Geometry: see drawing. Coordinates: mm, zero at the bounding-box minimum. Round coordinates to 2 decimals unless told otherwise and drop trailing zeros. Loops run counter-clockwise (first coordinate to the right, second up) from the corner with the lowest first, then second, coordinate; pieces in that order, holes last. Notation, with made-up numbers: (0.25, 74) -> (5.25, 74) arc R26 cw to (5.25, 100) -> close; hole circle Ø9 at (55, -37). An arc over 180 degrees is marked (long way). Answer in a Markdown table with one row per item.
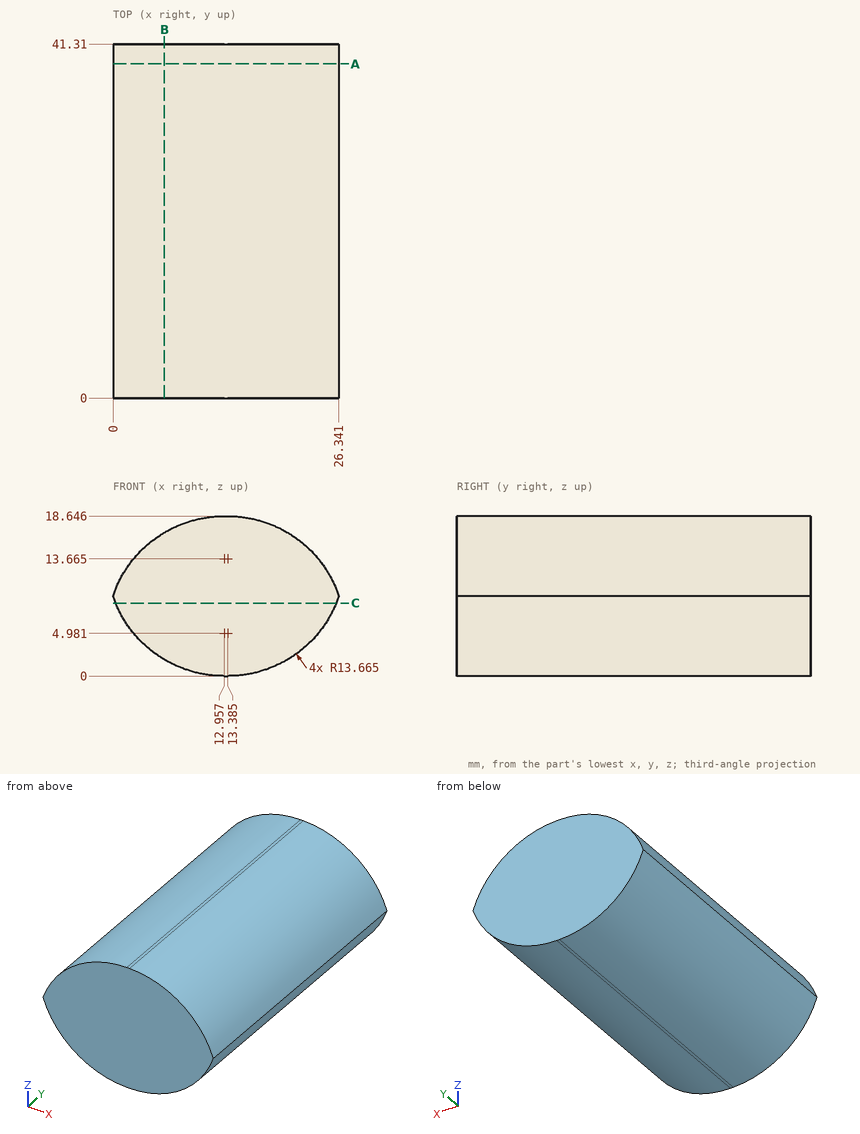
Item 1: Ray query, L1, parallel to X at y = 15, z = 12; L2, parallel to X at y = 8, z = 3.5 (1 decimal); L3, parallel to Z at x = 11.25, y = 5. Return the intervals inside material, ascending.
Ans:
| item | result |
|---|---|
| L1 | 1.23 to 25.11 |
| L2 | 3.8 to 22.5 |
| L3 | 0.11 to 18.54 |
Item 2: Section query C-C, the plane z = 8.5. Output: boundary loops of the cut face in (x, y) (1 decimal).
Ans:
| item | result |
|---|---|
| outline | (0.3, 0) -> (26, 0) -> (26, 41.3) -> (0.3, 41.3) -> close |
Item 3: First-contact query: P1, Ø4, axis at y = 30, z = 12, coming from the +X side (1 decimal); P2, Ø4, axis at x = 22.5, y = 28, coming from the +Z side; P3, Ø4, axis at x = 8, y = 21.5, coming from the -Z side. Flat tips, straight axial feed; report the tip coordinate or a pass-through.
Ans:
| item | result |
|---|---|
| P1 | x = 26.1 |
| P2 | z = 16.65 |
| P3 | z = 0.32 |
Item 4: Section query A-A, the plane y = 39. Output: boundary loops of the cut face in (x, z) (1 decimal).
Ans:
| item | result |
|---|---|
| outline | (0, 9.3) arc R13.7 ccw to (13, 0) -> (13.4, 0) arc R13.7 ccw to (26.3, 9.3) arc R13.7 ccw to (13.4, 18.6) -> (13, 18.6) arc R13.7 ccw to start |
Item 5: Section query B-B, the plane x = 6. Output: boundary loops of the cut face in (y, z), and give its area (3 significant figures).
Ans:
| item | result |
|---|---|
| outline | (0, 1.9) -> (41.31, 1.9) -> (41.31, 16.74) -> (0, 16.74) -> close |
| area | 613 mm2 |
